Work out the finished part from the listing and answer in its coordinate system (mm). Round coordinates to 2 decimals unless told otherwise and drop trailing zeros. Order: outer loops, then holes, each group sorted by start corner. A loop starts at its lowest first (then second) coordinate and runs counter-clockwise, first axis right, second up. Notation, with made-up numbers: (-28, 69.25) - (19, 69.25) arc R25 ccw to (19, 87.25) - close; hole circle Ø9 at (7.25, 73.25). An arc over 180 degrees is marked (long way). Answer in a Markdown table with one row per item.
from build123d import *

# Parameters (mm, degrees)
F1_DEPTH = 6.35
F2_D     = 8.8


# Not quite as in the source:
# - a length typed as a fraction of an inch, garbled in the dataset ("3 / 203.2 mm" for 3/8 in), is restored


with BuildPart() as f1:
    # F0 (on Front) → F1 (new body)
    with BuildSketch(Plane.XZ):
        Polygon((0, 114.3), (0, 0), (114.3, 0), (114.3, 38.1), (38.1, 38.1), (38.1, 114.3), align=None)
    extrude(amount=-F1_DEPTH)

    # F2 (through all)
    with Locations(Plane.XZ):
        with Locations((19.05, 95.25), (19.05, 57.15), (19.05, 19.05), (57.15, 19.05), (95.25, 19.05)):
            Hole(F2_D / 2)


solid = f1.part
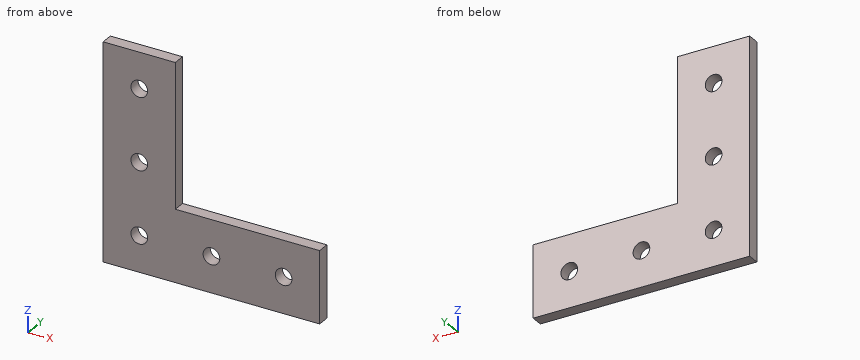
1) Find section B-B, the plane x = 95.25. Give the vertices of the cut face in (y, z).
Filled in:
| item | result |
|---|---|
| outline | (0, 0) - (6.35, 0) - (6.35, 14.65) - (0, 14.65) - close; (0, 23.45) - (6.35, 23.45) - (6.35, 38.1) - (0, 38.1) - close |
2) Find the intervals of material crossed by probe 1 along Z at (x, y) = (19.05, 2.5); probe 2 along Z at (x, y) = (57.15, 1.5); probe 3 along X at (y, z) = (4, 82), in increasing order. Write a range as from..to.
Filled in:
| item | result |
|---|---|
| probe 1 | z = 0..14.65, 23.45..52.75, 61.55..90.85, 99.65..114.3 |
| probe 2 | z = 0..14.65, 23.45..38.1 |
| probe 3 | x = 0..38.1 |
3) Find section D-D, the plane z = 19.05. Give the vertices of the cut face in (x, y), then the cut area to 3 significant figures.
Filled in:
| item | result |
|---|---|
| outline | (0, 0) - (14.65, 0) - (14.65, 6.35) - (0, 6.35) - close; (23.45, 0) - (52.75, 0) - (52.75, 6.35) - (23.45, 6.35) - close; (61.55, 0) - (90.85, 0) - (90.85, 6.35) - (61.55, 6.35) - close; (99.65, 0) - (114.3, 0) - (114.3, 6.35) - (99.65, 6.35) - close |
| area | 558 mm^2 |
4) Find section C-C, the plane y = 5.25. Give the vertices of the cut face in (x, z).
Filled in:
| item | result |
|---|---|
| outline | (0, 0) - (114.3, 0) - (114.3, 38.1) - (38.1, 38.1) - (38.1, 114.3) - (0, 114.3) - close; hole circle Ø8.8 at (19.05, 19.05); hole circle Ø8.8 at (19.05, 57.15); hole circle Ø8.8 at (19.05, 95.25); hole circle Ø8.8 at (57.15, 19.05); hole circle Ø8.8 at (95.25, 19.05) |
5) This flat-tipped pin is pushed along its axis until it touches: pin 1 (10 mm diameter, centred on x = 80.5, z = 44, fed in from +Y). Where does it stop, or does it pass through?
Filled in:
| item | result |
|---|---|
| pin 1 | passes through |
6) Find section A-A, the plane z = 57.15. Give the vertices of the cut face in (x, y), then the cut area to 3 significant figures.
Filled in:
| item | result |
|---|---|
| outline | (0, 0) - (14.65, 0) - (14.65, 6.35) - (0, 6.35) - close; (23.45, 0) - (38.1, 0) - (38.1, 6.35) - (23.45, 6.35) - close |
| area | 186 mm^2 |
